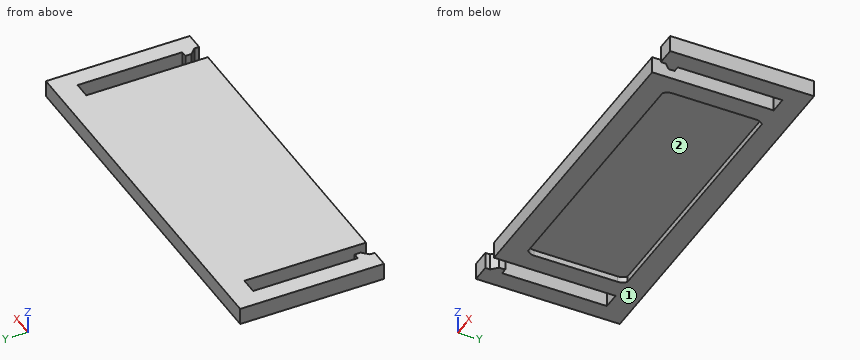
from build123d import *

# Parameters (mm, degrees)
SKETCH1_W                                = 62.4
SKETCH1_H                                = 23.902256307
SKETCH1_W_2                              = 2.8
SKETCH1_H_2                              = 17.402256307
BOSS_EXTRUDE1_DEPTH                      = 2.8
CUT_EXTRUDE1_DEPTH                       = 3.8
SKETCH4_W                                = 44.45
SKETCH4_H                                = 16.51
CUT_EXTRUDE2_DEPTH                       = 1
BOSS_EXTRUDE2_DEPTH                      = 1
MIRROR2_AT_THE_SECOND_PLANE_COPY_1_DEPTH = 1


with BuildPart() as part:
    # Sketch1 → Boss-Extrude1 (new body)
    with BuildSketch(Plane.XY):
        with Locations((-25.4, -14.348584576)):
            Rectangle(SKETCH1_W, SKETCH1_H)
        with Locations((-52.2, -14.798584576)):
            Rectangle(SKETCH1_W_2, SKETCH1_H_2, mode=Mode.SUBTRACT)
        with Locations((1.4, -14.798584576)):
            Rectangle(SKETCH1_W_2, SKETCH1_H_2, mode=Mode.SUBTRACT)
    extrude(amount=BOSS_EXTRUDE1_DEPTH)

    # Sketch2 → Cut-Extrude1 (cut, through all)
    with BuildSketch(Plane.XY.offset(2.8)):
        Polygon((-50.8, -23.499712729), (-52.6, -23.499712729), (-52.6, -24.499712729), (-53.6, -25.499712729), (-53.6, -26.299712729), (-50.8, -26.299712729), align=None)
    cut_extrude1 = extrude(amount=-CUT_EXTRUDE1_DEPTH, mode=Mode.SUBTRACT)

    # Mirror1: Cut-Extrude1 across plane
    add(cut_extrude1.mirror(Plane.ZY.offset(25.4)), mode=Mode.SUBTRACT)

    # Sketch4 → Cut-Extrude2 (cut)
    with BuildSketch(Plane(origin=(0, 0, 0), x_dir=(-1, 0, 0), z_dir=(0, 0, -1))):
        with Locations((25.4, -14.348584576)):
            Rectangle(SKETCH4_W, SKETCH4_H)
    extrude(amount=-CUT_EXTRUDE2_DEPTH, mode=Mode.SUBTRACT)

    # Sketch5 → Boss-Extrude2 (add)
    with BuildSketch(Plane(origin=(0, 0, 1), x_dir=(-1, 0, 0), z_dir=(0, 0, -1))):
        with BuildLine():
            Line((3.175, -6.093584576), (3.825, -6.093584576))
            ThreePointArc((3.825, -6.093584576), (3.346555815, -6.666862483), (3.175, -7.393584576))
            Line((3.175, -7.393584576), (3.175, -6.093584576))
        make_face()
    boss_extrude2 = extrude(amount=BOSS_EXTRUDE2_DEPTH)

    # Mirror2: Boss-Extrude2 across plane
    add(boss_extrude2.mirror(Plane.ZY.offset(25.4)))

    # Mirror2 at the second plane: Boss-Extrude2 across plane
    add(boss_extrude2.mirror(Plane.ZX.offset(-14.348584576)))

    # Mirror2 at the second plane copy 1 sketc → Mirror2 at the second plane copy 1 (add)
    with BuildSketch(Plane(origin=(-50.8, -28.697169151, 1), x_dir=(1, 0, 0), z_dir=(0, 0, -1))):
        with BuildLine():
            Line((3.175, -6.093584576), (3.825, -6.093584576))
            ThreePointArc((3.825, -6.093584576), (3.346555815, -6.666862483), (3.175, -7.393584576))
            Line((3.175, -7.393584576), (3.175, -6.093584576))
        make_face()
    extrude(amount=MIRROR2_AT_THE_SECOND_PLANE_COPY_1_DEPTH)


solid = part.part
Design review of the part built by this model. Coordinates are the model's own, in mm. Face numbers are marked on the shaded views. Give positions to 0.01 mm unless a question says otherwise; leave off trailing zeros. Loops run counter-clockwise (first coordinate to the right, second up) from the corner with the lowest first, then second, coordinate; pieces in that order, holes last. Notation, with made-up numbers: M -14.5,44.5 L -4.5,44.5 A19 ccw -4.5,81.5 Z; hole C 22,69.25 d1. An arc over 180 degrees is marked long. Write item = value, one per line.
Q1. We need section C-C (z = 1.75). Give the boundary of the cut face in (x, y).
Output values:
outline = M -56.6,-26.3 L -53.6,-26.3 L -53.6,-25.5 L -52.6,-24.5 L -52.6,-23.5 L -53.6,-23.5 L -53.6,-6.1 L -50.8,-6.1 L -50.8,-26.3 L 0,-26.3 L 0,-6.1 L 2.8,-6.1 L 2.8,-23.5 L 1.8,-23.5 L 1.8,-24.5 L 2.8,-25.5 L 2.8,-26.3 L 5.8,-26.3 L 5.8,-2.4 L -56.6,-2.4 Z
Q2. We need section B-B (x = -19). Give the boundary of the cut face in (y, z).
Output values:
outline = M -26.3,0 L -22.6,0 L -22.6,1 L -6.09,1 L -6.09,0 L -2.4,0 L -2.4,2.8 L -26.3,2.8 Z
Q3. We need section A-A (y = -14.25). Give the boundary of the cut face in (x, z) (3 decimals).
Output values:
outline = M -56.6,0 L -53.6,0 L -53.6,2.8 L -56.6,2.8 Z; M -50.8,0 L -47.625,0 L -47.625,1 L -3.175,1 L -3.175,0 L 0,0 L 0,2.8 L -50.8,2.8 Z; M 2.8,0 L 5.8,0 L 5.8,2.8 L 2.8,2.8 Z
Q4. To check wall thickness, follow line 1 (X direction, y = -13.5, z = 0.25) (3 decimals); line 2 (X direction, y = -23.25, z = 1.7); line 3 (Y direction, x = -9.5, z = 0.5). State the ranges of each line that lie inside material, in increasing order. Write a range as [from, to].
Output values:
line_1 = [-56.6, -53.6], [-50.8, -47.625], [-3.175, 0], [2.8, 5.8]
line_2 = [-56.6, -53.6], [-50.8, 0], [2.8, 5.8]
line_3 = [-26.3, -22.6], [-6.09, -2.4]
Q5. Draft analysis for pull direction X (two halves, no side actions). For the marked faces 1 and 2, state which applies: +X half, -X half, draft (parallel to the pull), parting line (faces both ways), or undercut.
Output values:
face_1 = draft
face_2 = undercut
Q6. Insertion check: pin 1 (5 mm diameter, centred on x = -24, y = -11, fed in from -Z); pin 2 (0.8 mm diameter, centred on x = -52, z = 1.5, fed in from -Y). Each pin has a flat end and moves straight along its axis. Give the tip position at first contact, or say it passes through.
Output values:
pin_1 = 1
pin_2 = -6.1
